from build123d import *

# Parameters (mm, degrees)
F0_W      = 48
F0_H      = 46
F1_DEPTH  = 16
F2_W      = 11
F2_H      = 25
F3_DEPTH  = 6
F5_DEPTH  = 10
F6_W      = 12
F6_H      = 5
F6_H_2    = 17
F7_DEPTH  = 20
F8_W      = 48
F8_H      = 15
F9_DEPTH  = 5
F10_W     = 7
F10_H     = 21
F11_DEPTH = 20
F13_DEPTH = 11
F14_R     = 2.5
F15_DEPTH = 59.501
F16_R     = 3
F17_DEPTH = 69.001
F18_R     = 2.25
F19_DEPTH = 26.001
F21_DEPTH = 2
F24_DEPTH = 14
F27_DEPTH = 14
F28_W     = 20
F28_H     = 4
F29_DEPTH = 8


with BuildPart() as f1:
    # F0 (on Top) → F1 (new body)
    with BuildSketch(Plane.XY):
        with Locations((0, -23)):
            Rectangle(F0_W, F0_H)
    extrude(amount=F1_DEPTH)

    # F2 (on Top) → F3 (join)
    with BuildSketch(Plane.XY):
        with Locations((0, 12.5)):
            Rectangle(F2_W, F2_H)
        Polygon((-19, 25), (-5.5, 25), (5.5, 25), (19, 25), (19, 30), (-19, 30), align=None)
    extrude(amount=F3_DEPTH)

    # F4 (on Top) → F5 (join)
    with BuildSketch(Plane.XY):
        Polygon((-45, 30), (0, 30), (45, 30), (45, 42), (24, 60), (-24, 60), (-45, 42), align=None)
    extrude(amount=F5_DEPTH)

    # F6 (on face) → F7 (join)
    with BuildSketch(Plane(origin=(0, 0, 0), x_dir=(1, 0, 0), z_dir=(0, 0, -1))):
        with Locations((-18, 31.5)):
            Rectangle(F6_W, F6_H)
        with Locations((18, 37.5)):
            Rectangle(F6_W, F6_H_2)
    extrude(amount=F7_DEPTH)

    # F8 (on face) → F9 (join)
    with BuildSketch(Plane(origin=(0, 0, 0), x_dir=(1, 0, 0), z_dir=(0, 0, -1))):
        with Locations((0, 38.5)):
            Rectangle(F8_W, F8_H)
    extrude(amount=F9_DEPTH)

    # F10 (on face) → F11 (join)
    with BuildSketch(Plane.XZ.offset(46)):
        with Locations((-11, 5.5)):
            Rectangle(F10_W, F10_H)
        with Locations((11, 5.5)):
            Rectangle(F10_W, F10_H)
    extrude(amount=F11_DEPTH)

    # F12 (on face) → F13 (cut)
    with BuildSketch(Plane.XY.offset(16)):
        Polygon((-11, 0), (-19, 0), (-19, -5), (-24, -5), (-24, -29), (-8, -29), (-8, -5), (-11, -5), align=None)
    extrude(amount=-F13_DEPTH, mode=Mode.SUBTRACT)

    # F14 (on face) → F15 (cut, through all)
    with BuildSketch(Plane(origin=(-14.5, 0, 0), x_dir=(0, -1, 0), z_dir=(-1, 0, 0))):
        with Locations((55, 10)):
            Circle(F14_R)
        with Locations((55, 1)):
            Circle(F14_R)
    extrude(amount=-F15_DEPTH, mode=Mode.SUBTRACT)

    # F16 (on face) → F17 (cut, through all)
    with BuildSketch(Plane(origin=(-24, 0, 0), x_dir=(0, -1, 0), z_dir=(-1, 0, 0))):
        with Locations((38.5, 1)):
            Circle(F16_R)
    extrude(amount=-F17_DEPTH, mode=Mode.SUBTRACT)

    # F18 (on face) → F19 (cut, through all)
    with BuildSketch(Plane.XY.offset(6)):
        with Locations((0, 6)):
            Circle(F18_R)
    extrude(amount=-F19_DEPTH, mode=Mode.SUBTRACT)

    # F20 (on face) → F21 (cut)
    with BuildSketch(Plane.XY.offset(6)):
        with BuildLine():
            Line((1.25, 0.464466), (1.25, 2.464466))
            ThreePointArc((1.25, 2.464466), (0, 9.75), (-1.25, 2.464466))
            Line((-1.25, 2.464466), (-1.25, 0.464466))
            Line((-1.25, 0.464466), (1.25, 0.464466))
        make_face()
    extrude(amount=-F21_DEPTH, mode=Mode.SUBTRACT)

    # F23 (on offset) → F24 (cut)
    with BuildSketch(Plane.YZ.offset(23)):
        Polygon((30, 0), (36.5, 0), (30, 7), align=None)
    extrude(amount=F24_DEPTH, mode=Mode.SUBTRACT)

    # F26 (on offset) → F27 (cut)
    with BuildSketch(Plane.YZ.offset(-23)):
        Polygon((30, 0), (36.5, 0), (30, 7), align=None)
    extrude(amount=-F27_DEPTH, mode=Mode.SUBTRACT)

    # F28 (on face) → F29 (join)
    with BuildSketch(Plane(origin=(0, 0, 0), x_dir=(1, 0, 0), z_dir=(0, 0, -1))):
        with Locations((0.275901, -55)):
            Rectangle(F28_W, F28_H)
    extrude(amount=F29_DEPTH)


solid = f1.part
Work out the finished part from the listing and answer in its coordinate system (mm). A direction names the side the tool comes from. Round coordinates to 2 decimals unless told otherwise and drop trailing zeros. Order: outer loops, then holes, each group sorted by start corner. A loop starts at its lowest first (then second) coordinate and runs counter-clockwise, first axis right, second up. Notation, with made-up numbers: M 88.5,73.5 L 131.5,73.5 A34 cw 131.5,111.5 Z; hole C 39,1.25 d4. An arc over 180 degrees is marked long. One line per item, written item: value.
Q1. Find section B-B on y = -55. Write down the section's boundary in (x, z).
Derived:
outline: M -14.5,-5 L -7.5,-5 L -7.5,-1.5 L -14.5,-1.5 Z; M -14.5,3.5 L -7.5,3.5 L -7.5,7.5 L -14.5,7.5 Z; M -14.5,12.5 L -7.5,12.5 L -7.5,16 L -14.5,16 Z; M 7.5,-5 L 14.5,-5 L 14.5,-1.5 L 7.5,-1.5 Z; M 7.5,3.5 L 14.5,3.5 L 14.5,7.5 L 7.5,7.5 Z; M 7.5,12.5 L 14.5,12.5 L 14.5,16 L 7.5,16 Z
Q2. For faces 4 (the face through (0, 53, -4)), 5 (the face through (0, 57, -4)), 6 (the face through (0, 19, 6)), determine the directions among +Z, -Z, +X, -X, +Y, -Y from which every point of the face is accessible in a straight line to the end or side of a thin tool.
Derived:
face 4: -Z, +X, -X
face 5: -Z, +X, -X, +Y
face 6: +Z, +X, -X
Q3. Flat-ended cylindrical pins translate along their axes: pin 1 (10 mm diameter, centred on x = -32.5, y = -34.5, fed in from +Z); pin 2 (8 mm diameter, centred on y = -55, z = 10, fed in from -X); pin 3 (9 mm diameter, centred on x = 21.5, y = 40.5, fed in from +Z); pin 4 (4 mm diameter, centred on y = -2.5, z = 10, fed in from -X). Find the tip coordinate at first contact, or state that the pin passes through.
Derived:
pin 1: through
pin 2: x = -14.5
pin 3: z = 10
pin 4: x = -24
Q4. Straight lines are drawn through the part: line 1 (Z direction, x = 10.25, y = -55); line 2 (Y direction, x = -22, z = 13.5); line 3 (Y direction, x = -7, z = -3.5). For each, find the intervals that lie inside material, in ascending order.
Derived:
line 1: -5 to -1.5, 3.5 to 7.5, 12.5 to 16
line 2: -46 to -29, -5 to 0
line 3: -46 to -31, 53 to 57
Q5. Find section A-A on y = 6. Write down the section's boundary in (x, z), then the cut area to 3 significant figures.
Derived:
outline: M -5.5,0 L -2.25,0 L -2.25,4 L -3.75,4 L -3.75,6 L -5.5,6 Z; M 2.25,0 L 5.5,0 L 5.5,6 L 3.75,6 L 3.75,4 L 2.25,4 Z
area: 33.0 mm²
Q6. Find section D-D on y = -38.5. Write down the section's boundary in (x, z).
Derived:
outline: M -24,-5 L 12,-5 L 12,-20 L 24,-20 L 24,-2 L -24,-2 Z; M -24,4 L 24,4 L 24,16 L -24,16 Z
Q7. Determine the mould class of faces 1 (the face through (14.5, -56, 5)), 2 (the face through (11, -66, 6)), 3 (the face through (-19, -2, 11)) for opening direction Y: released by +Y, released by -Y, zero draft, split by the parting line, or undercut.
Derived:
face 1: zero draft
face 2: released by -Y
face 3: undercut
Q8. Find section C-C on x = 31. Write down the section's boundary in (y, z), then the cut area to 3 significant figures.
Derived:
outline: M 30,7 L 36.5,0 L 54,0 L 54,10 L 30,10 Z
area: 217 mm²
